The listing builds one solid part. Answer for the finished solid, in the listing's coordinates (mm). Face numbers are marked on the shaded views. Round coordinates to 2 decimals unless told otherwise and drop trailing zeros. Order: outer loops, then holes, each group sorted by start corner. A loop starts at its lowest first (then second) coordinate and runs counter-clockwise, first axis right, second up. Notation, with made-up numbers: (86.5, 86) - (119.5, 86) arc R20 cw to (119.5, 97) - close; hole circle Ø1 at (72, -21). An arc over 180 degrees is marked (long way). Write item = value, one per line.
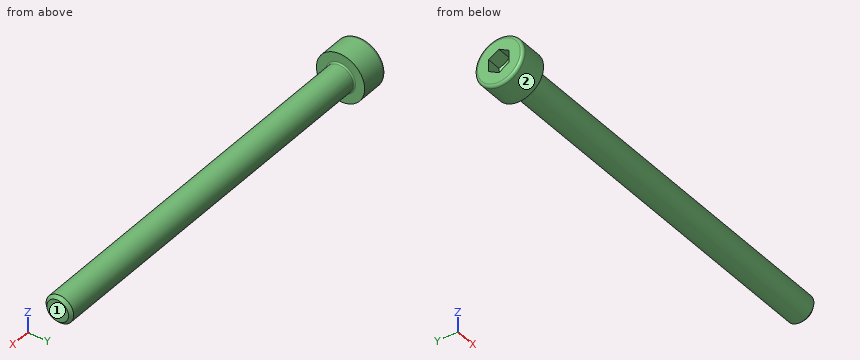
Autodesk Inventor part; units mm, degrees
ref_plane "Work Plane1" through (29, 0, 0) normal (0, -1, 0) x (1, 0, 0)
ref_plane "YZ Plane" through (0, 0, 0) normal (1, 0, 0) x (0, 1, 0)
ref_plane "XZ Plane" through (0, 0, 0) normal (0, 1, 0) x (-1, 0, 0)
sketch "Skizze1" plane through (0, 0, 0) normal (0, 0, 1) x (1, 0, 0)
  line L0 (-1, 0) -> (55, 0)
  line L1 (55, 0) -> (55, 2)
  line L2 (55, 2) -> (25, 2)
  line L3 (25, 2) -> (24.5705, 2)
  line L4 (24.5705, 2) -> (0, 2)
  line L5 (0, 2) -> (0, 3.5)
  line L6 (0, 3.5) -> (-4, 3.5)
  line L7 (-4, 3.5) -> (-4, 1.7321)
  line L8 (-4, 1.7321) -> (-2, 1.7321)
  line L9 (-2, 1.7321) -> (-1, 0)
  line L10 (-14.8, 0) -> (60.8, 0)
  line L11 (0, -0.7) -> (0, 4.2)
  line L12 (25, 2) -> (0, 2) construction
  dimension "d1" = 30
  dimension "d2" = 0.4295
  dimension "d3" = 4
  dimension "d4" = 2
  dimension "d5" = 60
  dimension "d6" = 4
  dimension "d7" = 4
  dimension "d8" = 3.4641
  dimension "d9" = 7
  dimension "d26" = 55
revolve "Körper" add sketch "Skizze1" angle 360 about axis through (-1, 0, 0) along (1, 0, 0)
sketch "Skizze2" plane through (-4, 0, 0) normal (-1, 0, 0) x (0, 0, 1)
  circle A0 centre (0, 0) radius 1.7321
  line L0 (0, -4.9) -> (0, 4.9)
  line L1 (-4.9, 0) -> (4.9, 0)
  line L2 (1.7321, 0) -> (0.866, -1.5)
  line L3 (0.866, -1.5) -> (-0.866, -1.5)
  line L4 (-0.866, -1.5) -> (-1.7321, 0)
  line L5 (-1.7321, 0) -> (-0.866, 1.5)
  line L6 (-0.866, 1.5) -> (0.866, 1.5)
  line L7 (0.866, 1.5) -> (1.7321, 0)
extrude "Loch" add sketch "Skizze2" against normal up to next contours L7 A0 | A0 L2 | L6 L0 A0 | A0 L0 L3 | L0 L6 A0 | A0 L3 L0 | L4 A0 | A0 L5
fillet "Rundung1" radius 0.4 1 edges at (-4, -3.5, 0)
thread "Gewinde"
chamfer "Fase1" distance 0.4294 distance2 0.4294 1 edges at (55, -2, 0) measured on face at (55, -0.3567, 0.5168)
ref_plane "Work Plane1" through (29, 0, 0) normal (0, -1, 0) x (1, 0, 0)
fillet "Fillet2" radius 0.2 1 edges at (0, -2, 0)
equation "\"d1\" = GEL"
equation "\"d3\" = KOH"
equation "\"d4\" = INTI"
equation "\"d6\" = GD"
equation "\"d7\" = BDM"
equation "\"d8\" = 1.1547 * SW"
equation "\"d9\" = KOD"
equation "\"d26\" = NLG"
equation "\"d30\" = R"
equation "\"d17\" = RR"
equation "\"d13\" = GEL"
equation "\"d15\" = -0.5 * SPD + 0.5 * GD"
equation "\"d16\" = GUL"
equation "\"GD\" = NND"
equation "\"NLG\" = 55"
equation "\"GEL\" = 30"
equation "\"KOD\" = 7"
equation "\"KOH\" = 4"
equation "\"INTI\" = 2"
equation "\"GAL\" = 0.61345 * PTC"
equation "\"GUL\" = 0.61345 * PTC"
equation "\"BDM\" = NND"
equation "\"SW\" = 3"
equation "\"RR\" = 0.4"
equation "\"SPD\" = NND - 1.2269 * PTC"
equation "\"R\" = 0.2"
equation "\"TOA\" = 30deg"
equation "\"GD1\" = THREADDIA - 1.2269 * PTC"
equation "\"THREADDIA\" = 4"
equation "\"FAWI\" = 45deg"
equation "\"ANG\" = 120deg"
equation "\"PTC\" = 0.7"
equation "\"NND\" = 4"
equation "\"E0\" = 1.155 * SW"
properties part number "DIN 912 - M4 x 55" material "Stahl, weich"
Q1. Section A-A on x = 30 is taken. Determine the outline of the cut face in (y, z).
Model answer:
outline = circle Ø4 at (0, 0)
Q2. Determine the mould class of the marked faces 1 and 2 for opening direction X: released by +X, released by -X, zero draft, split by the parting line, or undercut.
Model answer:
face_1 = released by +X
face_2 = zero draft
Q3. Flat-ended cylindrical pins translate along their axes: P1, Ø2, axis at x = 12.5, y = 1.5, coming from the +Z side; P2, Ø3, axis at x = 38.5, z = -2, coming from the -Y side; P3, Ø0.5, axis at x = -3, z = -0.5, coming from the +Y side. Find the tip coordinate at first contact, or state that the pin passes through.
Model answer:
P1 = 1.94
P2 = -1.94
P3 = 3.49
Q4. Find the intervals of material crossed by line 1 (X direction, y = -2.75, z = -1.5); line 2 (Z direction, x = 24.5, y = 1.25); line 3 (X direction, y = -1.25, z = 0), in increasing order. Write a range as from..to.
Model answer:
line_1 = -4..0
line_2 = -1.56..1.56
line_3 = -1.72..55
